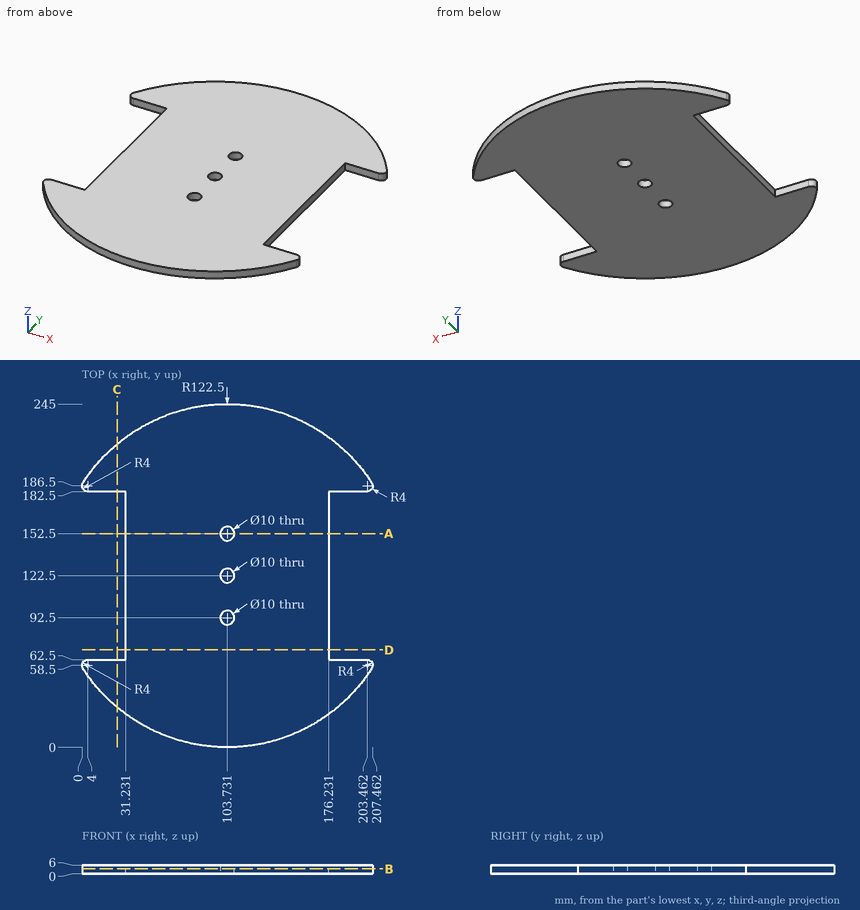
Geometry check sheet. Reference: drawing and pictorial views, mm from the part's lowest x, y, z. Give positions to 0.01 mm unless a question says otherwise; leave off trailing zeros. Order: outer loops, then holes, each group sorted by start corner. A loop starts at its lowest first (then second) coordinate and runs counter-clockwise, first axis right, second up. Notation, with made-up numbers: M 7.25,87.25 L 57.25,87.25 A25 cw 57.25,115.25 Z; hole C 87,78.5 d3. An arc over 180 degrees is marked long. Answer as CSV lines item,"result". Start each with the question number.
Item 1: Gauge pin test, flat ends, axial feed: P1, Ø3, axis at y = 129, z = 1.5, coming from the -X side; P2, Ø3, axis at y = 135.5, z = 1.5, coming from the +X side; P3, Ø6, axis at x = 103.73, y = 152.5, coming from the -Z side; P4, Ø2, axis at x = 146.5, z = 4.5, coming from the +Y side. Record the tip position at first contact, or that the pin passes through.
Item 2: Cross-section at D-D on y = 69.5. Enter the section's corners in (x, z), plus the area to 3 significant figures.
Item 3: Thickness scan on line 1 (X direction, y = 152.5, z = 3.35); line 2 (Y direction, x = 102, z = 1.4); line 3 (X direction, y = 107.5, z = 0.8). Record the ranges inside material, lowest first. Write a range as [from, to].
Item 4: Cross-section at A-A on y = 152.5. Enter the section's corners in (x, z), plus the area to 3 significant figures.
Item 5: Cross-section at C-C on x = 25. Enter the section's corners in (y, z), plus the area to 3 significant figures.
Item 6: Cross-section at B-B on z = 3.4. Enter the section's corners in (x, y).
Established:
1,P1,"stops at x = 31.23"
1,P2,"stops at x = 176.23"
1,P3,"passes through"
1,P4,"stops at y = 237.66"
2,outline,"M 31.23,0 L 176.23,0 L 176.23,6 L 31.23,6 Z"
2,area,"870 mm^2"
3,line 1,"x = [31.23, 98.73], [108.73, 176.23]"
3,line 2,"y = [0.01, 87.81], [97.19, 117.81], [127.19, 147.81], [157.19, 244.99]"
3,line 3,"x = [31.23, 176.23]"
4,outline,"M 31.23,0 L 98.73,0 L 98.73,6 L 31.23,6 Z; M 108.73,0 L 176.23,0 L 176.23,6 L 108.73,6 Z"
4,area,"810 mm^2"
5,outline,"M 28.65,0 L 62.5,0 L 62.5,6 L 28.65,6 Z; M 182.5,0 L 216.35,0 L 216.35,6 L 182.5,6 Z"
5,area,"406 mm^2"
6,outline,"M 0.63,56.34 A122.5 ccw 206.83,56.34 A4 ccw 203.46,62.5 L 176.23,62.5 L 176.23,182.5 L 203.46,182.5 A4 ccw 206.83,188.66 A122.5 ccw 0.63,188.66 A4 ccw 4,182.5 L 31.23,182.5 L 31.23,62.5 L 4,62.5 A4 ccw Z; hole C 103.73,92.5 d10; hole C 103.73,122.5 d10; hole C 103.73,152.5 d10"
